from build123d import *

# Parameters (mm, degrees)
ESBO_O1_R                = 6
RESSALTO_EXTRUS_O1_DEPTH = 45
ESBO_O2_R                = 18
RESSALTO_EXTRUS_O2_DEPTH = 10
ESBO_O3_R                = 6
RESSALTO_EXTRUS_O3_DEPTH = 25
ESBO_O4_W                = 4.529625907
ESBO_O4_H                = 11.468627296
ESBO_O4_W_2              = 6.059251814
ESBO_O4_H_2              = 15.612753126
CORTE_EXTRUS_O1_DEPTH    = 7


with BuildPart() as part:
    # Esboço1 → Ressalto-extrusão1 (new body)
    with BuildSketch(Plane.XY):
        with Locations(Location((0, 0, 0), (0, 0, 180))):
            Circle(ESBO_O1_R)
    extrude(amount=RESSALTO_EXTRUS_O1_DEPTH)

    # Esboço2 → Ressalto-extrusão2 (add)
    with BuildSketch(Plane.XY.offset(45)):
        Circle(ESBO_O2_R)
    extrude(amount=RESSALTO_EXTRUS_O2_DEPTH)

    # Esboço3 → Ressalto-extrusão3 (add)
    with BuildSketch(Plane.XY.offset(55)):
        with Locations((0, -8)):
            Circle(ESBO_O3_R)
    extrude(amount=RESSALTO_EXTRUS_O3_DEPTH)

    # Esboço4 → Corte-extrusão1 (cut)
    with BuildSketch(Plane(origin=(0, 0, 0), x_dir=(-1, 0, 0), z_dir=(0, 0, -1))):
        with Locations((-5.264812953, -0.433687587)):
            Rectangle(ESBO_O4_W, ESBO_O4_H)
        with Locations((6.029625907, -0.674625135)):
            Rectangle(ESBO_O4_W_2, ESBO_O4_H_2)
    extrude(amount=-CORTE_EXTRUS_O1_DEPTH, mode=Mode.SUBTRACT)


solid = part.part
Could you check a few things on this model? Use its own coordinates, in mm. A direction names the side the tool comes from. Round coordinates to 2 decimals unless told otherwise and drop trailing zeros. Loops run counter-clockwise (first coordinate to the right, second up) from the corner with the lowest first, then second, coordinate; pieces in that order, holes last. Notation, with made-up numbers: (-19.75, 32.5) - (-6.75, 32.5) arc R17 ccw to (-6.75, 47.5) - close; hole circle Ø6 at (-25, 43.5). An arc over 180 degrees is marked (long way). Write item = value, one per line.
1) I need wall thicknesses on line 1 along Z through (x, y) = (15, -1); line 2 along X through (y, z) = (-3, 29); line 3 along Z through (x, y) = (3, -11.5). Which ranges of each line are inside material? Lowest first, please. Write a range as from..to.
Computed:
line_1 = 45..55
line_2 = -5.2..5.2
line_3 = 45..80
2) Imagine slicing it at A-A (y = 0). Please give me the cut outline in (x, z).
Computed:
outline = (-18, 45) - (-6, 45) - (-6, 7) - (-3, 7) - (-3, 0) - (3, 0) - (3, 7) - (6, 7) - (6, 45) - (18, 45) - (18, 55) - (-18, 55) - close
3) Imagine slicing it at D-D (y = -4). Please give me the cut outline in (x, z), and give its area (3 significant figures).
Computed:
outline = (-17.55, 45) - (-4.47, 45) - (-4.47, 7) - (-3, 7) - (-3, 0) - (3, 0) - (3, 7) - (4.47, 7) - (4.47, 45) - (17.55, 45) - (17.55, 55) - (4.47, 55) - (4.47, 80) - (-4.47, 80) - (-4.47, 55) - (-17.55, 55) - close
area = 956 mm2
4) Imagine slicing it at C-C (z = 16.5). Please give me the cut outline in (x, y).
Computed:
outline = circle Ø12 at (0, 0)
5) Imagine slicing it at B-B (x = 0). Please give me the cut outline in (y, z), and give its area (3 significant figures).
Computed:
outline = (-18, 45) - (-6, 45) - (-6, 0) - (6, 0) - (6, 45) - (18, 45) - (18, 55) - (-2, 55) - (-2, 80) - (-14, 80) - (-14, 55) - (-18, 55) - close
area = 1,200 mm2
6) I'm going to push flat-ended pins straight in: P1, Ø3, axis at y = 7, z = 14, coming from the +X side; P2, Ø1.5, axis at y = 1, z = 43, coming from the -X side; P3, Ø1, axis at x = 6, y = 0, coming from the +Z side. Where does each tip first touch, or does it pass through?
Computed:
P1 = 2.4
P2 = -5.99
P3 = 55
7) On a 3-axis mill with a long thin cutter (end or side, diameter ignored), from which of +Z, -Z, +X, -X, +Y, -Y can I reach the whole of each face in a straight line? I mean faces 1 (the cylindrical face through (-2.769, 5.323, 22.185)), 2 (the flat face through (4, 0, 7)), 3 (the cylindrical face through (-0.78, -2.05, 67.32)). Say none if no direction works.
Computed:
face_1 = -Z
face_2 = -Z, +X, +Y, -Y
face_3 = +Z
